Source: CAD feature listing. Evaluate the final solid. Frame: model axes, mm. Give positions to 0.01 mm unless a question says otherwise; leave off trailing zeros. Loops run counter-clockwise (first coordinate to the right, second up) from the corner with the lowest first, then second, coordinate; pieces in that order, holes last.
```python
from build123d import *

# Parameters (mm, degrees)
SKETCH1_R                   = 30
BOSS_EXTRUDE1_DEPTH         = 4
CUT_EXTRUDE3_START          = 4
SKETCH1_4_W                 = 3.8
SKETCH1_4_H                 = 6
SKETCH1_4_H_2               = 8
SKETCH1_4_W_2               = 6
SKETCH1_4_H_3               = 3.8
SKETCH1_4_W_3               = 8
CUT_EXTRUDE3_DEPTH          = 5
CUT_EXTRUDE5_START          = 4
SKETCH1_5_R                 = 1.5
CUT_EXTRUDE5_DEPTH          = 5
CIRPATTERN2_COUNT           = 4
CIRPATTERN2_START           = 4
CIRPATTERN2_COPY_1_SKETCH_R = 1.5
CIRPATTERN2_COPY_1_DEPTH    = 5
CIRPATTERN2_COPY_2_SKETCH_R = 1.5
CIRPATTERN2_COPY_2_DEPTH    = 5
CIRPATTERN2_COPY_3_SKETCH_R = 1.5
CIRPATTERN2_COPY_3_DEPTH    = 5
CIRPATTERN3_COUNT           = 2


with BuildPart() as part:
    # Sketch1 → Boss-Extrude1 (new body)
    with BuildSketch(Plane(origin=(0, 0, 0), x_dir=(1, 0, 0), z_dir=(0, 1, 0))):
        Circle(SKETCH1_R)
    extrude(amount=BOSS_EXTRUDE1_DEPTH)

    # Sketch1<4> → Cut-Extrude3 (cut, through all)
    with BuildSketch(Plane(origin=(0, 0, 0), x_dir=(1, 0, 0), z_dir=(0, 1, 0)).offset(CUT_EXTRUDE3_START)):
        with Locations((0, 3)):
            Rectangle(SKETCH1_4_W, SKETCH1_4_H)
        with Locations((0, 18.5)):
            Rectangle(SKETCH1_4_W, SKETCH1_4_H_2)
        with Locations((3, 0)):
            Rectangle(SKETCH1_4_W_2, SKETCH1_4_H_3)
        with Locations((22.04, 0)):
            Rectangle(SKETCH1_4_W_3, SKETCH1_4_H_3)
    cut_extrude3 = extrude(amount=-CUT_EXTRUDE3_DEPTH, mode=Mode.SUBTRACT)

    # Sketch1<5> → Cut-Extrude5 (cut, through all)
    with BuildSketch(Plane(origin=(0, 0, 0), x_dir=(1, 0, 0), z_dir=(0, 1, 0)).offset(CUT_EXTRUDE5_START)):
        with Locations((8.34, 23.4)):
            Circle(SKETCH1_5_R)
    cut_extrude5 = extrude(amount=-CUT_EXTRUDE5_DEPTH, mode=Mode.SUBTRACT)

    # Mirror1: Cut-Extrude5 across plane
    add(cut_extrude5.mirror(Plane(origin=(0, 0, 0), x_dir=(0, 0, 1), z_dir=(1, 0, 0))), mode=Mode.SUBTRACT)

    # CirPattern2: Cut-Extrude5 ×4 about axis
    cirpattern2_axis = Axis((0, 0, 0), (0, 1, 0))
    for i in range(1, CIRPATTERN2_COUNT):
        add(cut_extrude5.rotate(cirpattern2_axis, i * 360 / CIRPATTERN2_COUNT), mode=Mode.SUBTRACT)

    # CirPattern2 copy 1 sketch → CirPattern2 copy 1 (cut, through all)
    with BuildSketch(Plane.ZX.offset(CIRPATTERN2_START)):
        with Locations((8.34, -23.4)):
            Circle(CIRPATTERN2_COPY_1_SKETCH_R)
    extrude(amount=-CIRPATTERN2_COPY_1_DEPTH, mode=Mode.SUBTRACT)

    # CirPattern2 copy 2 sketch → CirPattern2 copy 2 (cut, through all)
    with BuildSketch(Plane(origin=(0, 0, 0), x_dir=(1, 0, 0), z_dir=(0, 1, 0)).offset(CIRPATTERN2_START)):
        with Locations((8.34, -23.4)):
            Circle(CIRPATTERN2_COPY_2_SKETCH_R)
    extrude(amount=-CIRPATTERN2_COPY_2_DEPTH, mode=Mode.SUBTRACT)

    # CirPattern2 copy 3 sketch → CirPattern2 copy 3 (cut, through all)
    with BuildSketch(Plane(origin=(0, 0, 0), x_dir=(0, 0, -1), z_dir=(0, 1, 0)).offset(CIRPATTERN2_START)):
        with Locations((8.34, -23.4)):
            Circle(CIRPATTERN2_COPY_3_SKETCH_R)
    extrude(amount=-CIRPATTERN2_COPY_3_DEPTH, mode=Mode.SUBTRACT)

    # CirPattern3: Cut-Extrude3 ×2 about axis
    cirpattern3_axis = Axis((0, 0, 0), (0, 1, 0))
    for i in range(1, CIRPATTERN3_COUNT):
        add(cut_extrude3.rotate(cirpattern3_axis, i * 360 / CIRPATTERN3_COUNT), mode=Mode.SUBTRACT)


solid = part.part
```
(1) Ray query, line 1 along Z through (x, y) = (-8, 0.75); line 2 along Z through (x, y) = (-24, 2.45); line 3 along Z through (x, y) = (8.34, 1.3). Return the intervals inside material, ascending.
A:
line 1: z = -28.91 to -24.86, -21.94 to 21.94, 24.86 to 28.91
line 2: z = -18 to -9.71, -6.97 to -1.9, 1.9 to 6.97, 9.71 to 18
line 3: z = -28.82 to -24.9, -21.9 to 21.9, 24.9 to 28.82
(2) Section D-D, the plane x = -23.4. Return the cut outline in (y, z).
A:
outline: (0, -18.77) - (4, -18.77) - (4, -9.84) - (0, -9.84) - close; (0, -6.84) - (4, -6.84) - (4, -1.9) - (0, -1.9) - close; (0, 1.9) - (4, 1.9) - (4, 6.84) - (0, 6.84) - close; (0, 9.84) - (4, 9.84) - (4, 18.77) - (0, 18.77) - close
(3) Section B-B, the plane x = 8.34. Return the cut outline in (y, z).
A:
outline: (0, -28.82) - (4, -28.82) - (4, -24.9) - (0, -24.9) - close; (0, -21.9) - (4, -21.9) - (4, 21.9) - (0, 21.9) - close; (0, 24.9) - (4, 24.9) - (4, 28.82) - (0, 28.82) - close
(4) First-contact query: pin 1 (2 mm diameter, centred on x = 22.5, y = 2, fed in from -Z); pin 2 (2 mm diameter, centred on x = -20.5, y = 2, fed in from -Z). Flat tips, straight axial feed; report the tip coordinate or a pass-through.
A:
pin 1: stops at z = -20.92
pin 2: stops at z = -22.8
(5) Mould query, pull axis X, two halves, no side actions, for faces 1 (the flat face through (22, 2, 1.9)), 2 (the flat face through (1.9, 2, -18)), 3 (the cylindrical face through (-29.97, 1.97, -1.32)). Classes: pulls with the +X half, pulls with the -X half, needs draft (parallel to the pull), parting line crosses it, or undercut.
A:
face 1: undercut
face 2: undercut
face 3: parting line crosses it
(6) Section A-A, the plane z = 0. Return the cut outline in (x, y).
A:
outline: (-30, 0) - (-26.04, 0) - (-26.04, 4) - (-30, 4) - close; (-18.04, 0) - (-6, 0) - (-6, 4) - (-18.04, 4) - close; (6, 0) - (18.04, 0) - (18.04, 4) - (6, 4) - close; (26.04, 0) - (30, 0) - (30, 4) - (26.04, 4) - close
(7) Section C-C, the plane z = 19. Return the cut outline in (x, y).
A:
outline: (-23.22, 0) - (-1.9, 0) - (-1.9, 4) - (-23.22, 4) - close; (1.9, 0) - (23.22, 0) - (23.22, 4) - (1.9, 4) - close
